Verification items for the finished model (mm, model axes). A direction names the side the tool comes from. Give positions to 0.01 mm unless a question says otherwise; leave off trailing zeros. Write each loop counter-clockwise with the first axis right and the second up, starting at its lowest first coordinate (ties: lowest second). Pieces come first, ordered by that corner, then holes. Notation, with made-up numbers: (12.5, 17.25) -> (47.5, 17.25) arc R13 cw to (47.5, 38.25) -> close; hole circle Ø7 at (-34.5, 46.25). An arc over 180 degrees is marked (long way). Answer as CSV lines item,"result".
```python
from build123d import *

# Parameters (mm, degrees)
SKETCH1_R           = 18.5
BOSS_EXTRUDE1_DEPTH = 56.6928
FILLET3_R           = 0.1
SKETCH2_R           = 6
BOSS_EXTRUDE2_DEPTH = 3.175
FILLET2_R           = 1.5875
SKETCH5_R           = 3
BOSS_EXTRUDE3_DEPTH = 15
CUT_EXTRUDE1_START  = -14
CUT_EXTRUDE1_DEPTH  = 14
SKETCH7_R           = 1.5
CUT_EXTRUDE2_DEPTH  = 10


with BuildPart() as part:
    # Sketch1 → Boss-Extrude1 (new body)
    with BuildSketch(Plane.XY):
        Circle(SKETCH1_R)
    extrude(amount=BOSS_EXTRUDE1_DEPTH)

    # Fillet3
    fillet3_edges = [part.edges().sort_by_distance(p)[0] for p in [
        (-18.5, 0, 56.6928),
    ]]
    fillet(fillet3_edges, radius=FILLET3_R)

    # Sketch2 → Boss-Extrude2 (add)
    with BuildSketch(Plane.XY.offset(56.6928)):
        Circle(SKETCH2_R)
    extrude(amount=BOSS_EXTRUDE2_DEPTH)

    # Fillet2
    fillet2_edges = [part.edges().sort_by_distance(p)[0] for p in [
        (-6, 0, 59.8678),
    ]]
    fillet(fillet2_edges, radius=FILLET2_R)

    # Sketch5 → Boss-Extrude3 (add)
    with BuildSketch(Plane.XY.offset(59.8678)):
        Circle(SKETCH5_R)
    extrude(amount=BOSS_EXTRUDE3_DEPTH)

    # Sketch6 → Cut-Extrude1 (cut)
    with BuildSketch(Plane.XY.offset(74.8678).offset(CUT_EXTRUDE1_START)):
        with BuildLine():
            Line((-1.658312395, 2.5), (1.658312395, 2.5))
            ThreePointArc((1.658312395, 2.5), (0, 3), (-1.658312395, 2.5))
        make_face()
    extrude(amount=CUT_EXTRUDE1_DEPTH, mode=Mode.SUBTRACT)

    # Sketch7 → Cut-Extrude2 (cut)
    with BuildSketch(Plane.XY.offset(56.6928)):
        with Locations((0, 15.5)):
            Circle(SKETCH7_R)
        with Locations((13.423393759, 7.75)):
            Circle(SKETCH7_R)
        with Locations((13.423393759, -7.75)):
            Circle(SKETCH7_R)
        with Locations((0, -15.5)):
            Circle(SKETCH7_R)
        with Locations((-13.423393759, -7.75)):
            Circle(SKETCH7_R)
        with Locations((-13.423393759, 7.75)):
            Circle(SKETCH7_R)
    extrude(amount=-CUT_EXTRUDE2_DEPTH, mode=Mode.SUBTRACT)


solid = part.part
```
1) Scan lines: line 1 along Y through (x, z) = (0, 52.25); line 2 along X through (y, z) = (-7, 50); line 3 along Y through (x, z) = (2, 26.5). Record each from-to range of solid material in increasing order.
Reported:
line 1,"-18.5 to -17, -14 to 14, 17 to 18.5"
line 2,"-17.12 to -14.72, -12.12 to 12.12, 14.72 to 17.12"
line 3,"-18.39 to 18.39"
2) Draft check along Y on faces 4 (the flat face through (-4.35, 4.35, 56.693)), 5 (the cylindrical face through (-0.65, -2.93, 67.26)), 6 (the flat face through (0, 16, 46.693)). Enter one of: +Y half, -Y half, draft (parallel to the pull), parting line (faces both ways), or undercut.
Reported:
face 4,"draft"
face 5,"parting line"
face 6,"undercut"
3) Section check C-C (z = 41.5). Record the boundary of the cut face in (x, y), and give its area (3 significant figures).
Reported:
outline,"circle Ø37 at (0, 0)"
area,"1,080 mm²"
4) Tool access check on faces 1 (the flat face through (0, 2.5, 68)), 2 (the flat face through (0, 0, 0)), 3 (the flat face through (-13, -8, 46.693)). Record the directions out of +Z, -Z, +X, -X, +Y, -Y that give a thin tool (end or side, any length) a straight path to the whole face; none if there is none.
Reported:
face 1,"+Z, +X, -X, +Y"
face 2,"-Z, +X, -X, +Y, -Y"
face 3,"+Z"
5) Depth check by flat-ended pin: pin 1 (12 mm diameter, centred on x = 13, z = 20.5, fed in from -Y); pin 2 (2 mm diameter, centred on x = -4.5, y = 10, fed in from -Z); pin 3 (1 mm diameter, centred on x = -0.5, z = 67.5, fed in from +Y); pin 4 (2.5 mm diameter, centred on x = 13, y = 7.5, fed in from +Z). Enter the tip coordinate at first touch or a pass-through.
Reported:
pin 1,"y = -17.12"
pin 2,"z = 0"
pin 3,"y = 2.5"
pin 4,"z = 56.69"
